Drawing for the job (mm, zero at the part's lowest x, y, z). A direction names the side the tool comes from. Round coordinates to 2 decimals unless told otherwise and drop trailing zeros. Loops run counter-clockwise (first coordinate to the right, second up) from the corner with the lowest first, then second, coordinate; pieces in that order, holes last. Notation, with made-up numbers: (64.25, 65.5) - (106.25, 65.5) arc R25 ccw to (106.25, 88.5) - close; hole circle Ø7 at (62.5, 45). An arc over 180 degrees is marked (long way). Put each result on its own line as item: value.
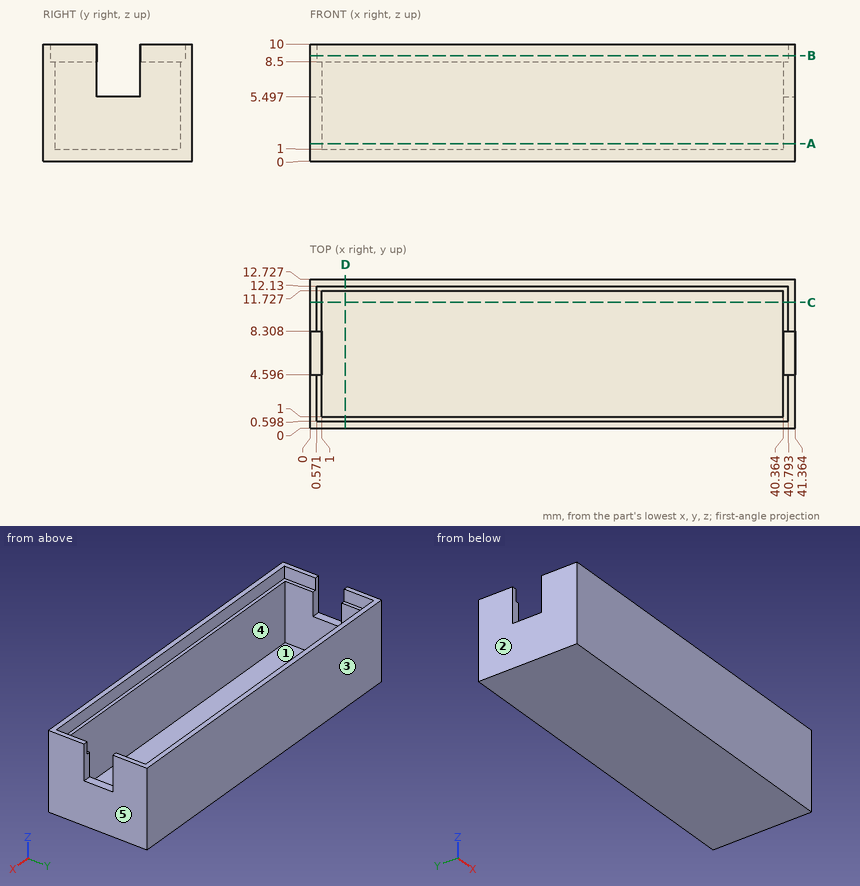
1. Band-saw the part on B-B (z = 9). List the corners of the cut face in (x, y).
A:
outline: (0, 0) - (41.36, 0) - (41.36, 4.6) - (40.79, 4.6) - (40.79, 0.6) - (0.57, 0.6) - (0.57, 4.6) - (0, 4.6) - close; (0, 8.31) - (0.57, 8.31) - (0.57, 12.13) - (40.79, 12.13) - (40.79, 8.31) - (41.36, 8.31) - (41.36, 12.73) - (0, 12.73) - close
2. Band-saw the part on D-D (x = 3). List the corners of the cut face in (y, z).
A:
outline: (0, 0) - (12.73, 0) - (12.73, 10) - (12.13, 10) - (12.13, 8.5) - (11.73, 8.5) - (11.73, 1) - (1, 1) - (1, 8.5) - (0.6, 8.5) - (0.6, 10) - (0, 10) - close
3. Probe line 1 along X through (y, z) = (6.5, 2.25); line 2 along Y through (x, z) = (17, 2.75); line 3 along X through (y, z) = (1.25, 8.75). List the from-to ranges inside material, lowest first. Write a range as [from, to].
A:
line 1: x = [0, 1], [40.36, 41.36]
line 2: y = [0, 1], [11.73, 12.73]
line 3: x = [0, 0.57], [40.79, 41.36]
4. Pin check, flat tips, straight feed: P1, Ø1.6, axis at y = 10, z = 9, coming from the -X side; P2, Ø1.9, axis at x = 17.5, y = 9.5, coming from the +Z side; P3, Ø4.5, axis at x = 22, y = 3, coming from the +Z side. Stop position of each tip, or through.
A:
P1: stops at x = 0
P2: stops at z = 1
P3: stops at z = 8.5
5. Tool access for the marked faces 4 and 5: list every direction of +Z, -Z, +X, -X, +Y, -Y with a clear straight run to the whole face (end or side of a thin tool).
A:
face 4: +Z
face 5: +Z, -Z, +X, +Y, -Y
6. Band-saw the part on A-A (z = 1.5). List the corners of the cut face in (x, y).
A:
outline: (0, 0) - (41.36, 0) - (41.36, 12.73) - (0, 12.73) - close; hole (1, 1) - (40.36, 1) - (40.36, 11.73) - (1, 11.73) - close
7. Two-plate mould, pull along Y, no slides. Class the marked faces 1, 2 and 3: pulls with the +Y half, pulls with the -Y half, needs draft (parallel to the pull), parting line crosses it, or undercut.
A:
face 1: undercut
face 2: needs draft
face 3: pulls with the +Y half
8. Band-saw the part on C-C (y = 10.75). List the corners of the cut face in (x, z).
A:
outline: (0, 0) - (41.36, 0) - (41.36, 10) - (40.79, 10) - (40.79, 8.5) - (40.36, 8.5) - (40.36, 1) - (1, 1) - (1, 8.5) - (0.57, 8.5) - (0.57, 10) - (0, 10) - close
